Autodesk Inventor part; units mm, degrees
ref_plane "YZ Plane" through (0, 0, 0) normal (1, 0, 0) x (0, 1, 0)
ref_plane "XZ Plane" through (0, 0, 0) normal (0, 1, 0) x (-1, 0, 0)
ref_plane "XY Plane" through (0, 0, 0) normal (0, 0, 1) x (1, 0, 0)
sketch "Sketch1" plane through (0, 0, 0) normal (0, 0, 1) x (1, 0, 0)
  line L0 (0, 0) -> (10, 0)
  line L1 (10, 0) -> (10, 10)
  line L2 (10, 10) -> (0, 10)
  line L3 (0, 10) -> (0, 0)
  dimension "d0" = 10
  dimension "d1" = 10
extrude "Plate1" add sketch "Sketch1" along normal blind 1
sketch "Sketch2" plane through (10, 1, 0) normal (0, -1, 0) x (1, 0, 0)
  line L0 (-10, 0) -> (0, 0)
  line L1 (0, 0) -> (0, 10)
  line L2 (0, 10) -> (-10, 10)
  line L3 (-10, 10) -> (-10, 0)
edge flange "Flange1" height 10 angle 90 thickness 1 bend radius 0.3 thickness toward (0, -1, 0) relief tear relief width 1 relief depth 0.5 edges at (5, 0, 1) wall of the first edge with corners at (0, 1, 0) (10, 1, 0) (10, 1, 10) (0, 1, 10)
bend "Bend1"
corner "Corner1"
sketch "Sketch3" plane through (0, 0, 0) normal (0, 0, -1) x (-1, 0, 0)
  circle A0 centre (-5, 7) radius 1.75
  line L0 (-10, 10) -> (0, 10)
  line L1 (-10, 1) -> (0, 1)
  point P0 (0, 0)
  point P1 (-5, 10)
  dimension "d13" = 3.5
  dimension "d14" = 6
extrude "Extrusion1" cut sketch "Sketch3" against normal blind 10
sketch "Sketch4" plane through (0, 0, 10) normal (0, -1, 0) x (1, 0, 0)
  circle A0 centre (5, -3) radius 1.75
  line L0 (0, -9) -> (10, -9)
  line L1 (0, 0) -> (10, 0)
  point P0 (0, -10)
  point P1 (5, 0)
  dimension "d17" = 3.5
  dimension "d18" = 6
extrude "Extrusion2" cut sketch "Sketch4" against normal blind 10
equation "\"d2\" = 厚度"
equation "\"d3\" = 折彎離隙寬度"
equation "\"d4\" = 折彎離隙深度"
equation "\"d5\" = 最小剩餘"
equation "\"d6\" = 轉移半徑"
equation "\"d10\" = 轉角離隙大小"
equation "\"d11\" = 間隙大小"
equation "\"d12\" = Jacobi半徑大小"
equation "\"折彎半徑\" = 厚度"
equation "\"折彎離隙寬度\" = 厚度"
equation "\"折彎離隙深度\" = 0.5 * 厚度"
equation "\"轉角離隙大小\" = 4 * 厚度"
equation "\"最小剩餘\" = 2 * 厚度"
equation "\"轉移半徑\" = 折彎半徑"
equation "\"Jacobi半徑大小\" = 折彎半徑"
equation "\"間隙大小\" = 厚度"
properties part number "joint"
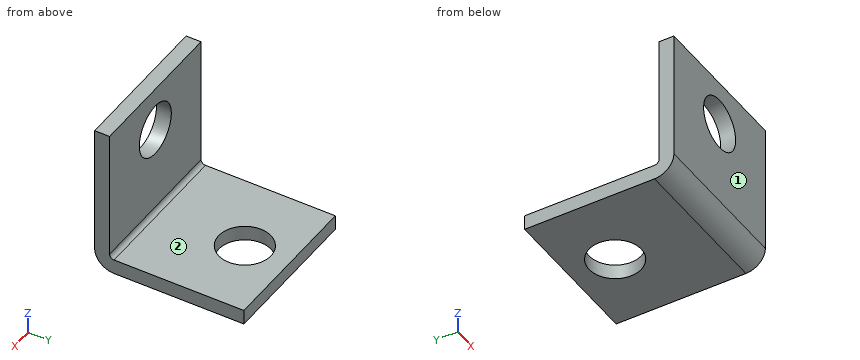
Verification items for the finished model (mm, model axes). Face numbers are marked on the shaded views. A direction names the side the tool comes from. Coordinates: 2 decimals unless noted, no trailing zeros. Loops run counter-clockwise (first coordinate to the right, second up) from the corner with the lowest first, then second, coordinate; pieces in that order, holes last. Notation, with made-up numbers: (80.25, 62.25) -> (106.25, 62.25) arc R25 cw to (106.25, 78.25) -> close; hole circle Ø1 at (-40, 15.25). An arc over 180 degrees is marked (long way). Write each question's results on one line, items separated by ' | '.
Item 1: Section check B-B, the plane y = 7. Enter the section's corners in (x, z).
Found:
outline: (0, 0) -> (3.25, 0) -> (3.25, 1) -> (0, 1) -> close; (6.75, 0) -> (10, 0) -> (10, 1) -> (6.75, 1) -> close
Item 2: Section check A-A, the plane x = 5. Enter the section's corners in (y, z), plus the area to 3 significant figures.
Found:
outline: (0, 1.3) arc R1.3 ccw to (1.3, 0) -> (5.25, 0) -> (5.25, 1) -> (1.3, 1) arc R0.3 cw to (1, 1.3) -> (1, 5.25) -> (0, 5.25) -> close; (0, 8.75) -> (1, 8.75) -> (1, 10) -> (0, 10) -> close; (8.75, 0) -> (10, 0) -> (10, 1) -> (8.75, 1) -> close | area: 11.7 mm2
Item 3: Material ranges on L1, parallel to Z at x = 7.5, y = 8.5; L2, parallel to Y at x = 5, z = 0.5, recorded low to high.
Found:
L1: z = 0 to 1 | L2: y = 0.28 to 5.25, 8.75 to 10
Item 4: Tool access check on the marked faces 1 and 2. Record the directions out of +Z, -Z, +X, -X, +Y, -Y that give a thin tool (end or side, any length) a straight path to the whole face; none if there is none.
Found:
face 1: +Z, -Z, +X, -X, -Y | face 2: +Z, +X, -X, +Y
Item 5: Gauge pin test, flat ends, axial feed: pin 1 (4 mm diameter, centred on x = 5, y = 7, fed in from -Z); pin 2 (5.5 mm diameter, centred on x = 5, z = 7, fed in from +Y); pin 3 (2.5 mm diameter, centred on x = 5.5, y = 4, fed in from +Z). Record the tip position at first contact, or that the pin passes through.
Found:
pin 1: stops at z = 0 | pin 2: stops at y = 1 | pin 3: stops at z = 1
Item 6: Section check D-D, the plane x = 7. Enter the section's corners in (y, z).
Found:
outline: (0, 1.3) arc R1.3 ccw to (1.3, 0) -> (10, 0) -> (10, 1) -> (1.3, 1) arc R0.3 cw to (1, 1.3) -> (1, 10) -> (0, 10) -> close
